from build123d import *

# Parameters (mm, degrees)
F1_W      = 129
F1_H      = 100.5
F1_W_2    = 127
F1_H_2    = 98.5
F2_DEPTH  = 6
F3_W      = 129
F3_H      = 100.5
F3_W_2    = 127
F3_H_2    = 90.5
F4_DEPTH  = 22
F6_DEPTH  = 17
F7_R      = 1.4
F8_DEPTH  = 7.9
F9_R      = 1.4
F10_DEPTH = 5
F11_W     = 127
F11_H     = 98.5
F11_W_2   = 115
F11_H_2   = 86
F12_DEPTH = 5


with BuildPart() as f2:
    # F1 (on Front) → F2 (new body)
    with BuildSketch(Plane.XZ):
        with Locations((1, -2.75)):
            Rectangle(F1_W, F1_H)
        with Locations((1, -2.75)):
            Rectangle(F1_W_2, F1_H_2, mode=Mode.SUBTRACT)
    extrude(amount=F2_DEPTH)

    # F3 (on Front) → F4 (join)
    with BuildSketch(Plane.XZ):
        with Locations((1, -2.75)):
            Rectangle(F3_W, F3_H)
        with Locations((1, -2.75)):
            Rectangle(F3_W_2, F3_H_2, mode=Mode.SUBTRACT)
    extrude(amount=-F4_DEPTH)

    # F5 (on face) → F6 (join)
    with BuildSketch(Plane(origin=(0, 22, 0), x_dir=(-1, 0, 0), z_dir=(0, 1, 0))):
        Polygon((3.5, -66.5), (63.5, -66.5), (63.5, -53), (55.5, -53), (55.5, -61.5), (11.5, -61.5), (11.5, -53), (3.5, -53), align=None)
    extrude(amount=-F6_DEPTH)

    # F7 (on face) → F8 (cut)
    with BuildSketch(Plane.XY.offset(47.5)):
        with Locations((-27.5, 16.5)):
            Circle(F7_R)
        with Locations((31.5, 16.5)):
            Circle(F7_R)
    extrude(amount=-F8_DEPTH, mode=Mode.SUBTRACT)

    # F9 (on face) → F10 (cut)
    with BuildSketch(Plane(origin=(0, 0, -66.5), x_dir=(1, 0, 0), z_dir=(0, 0, -1))):
        with Locations((-27.5, -16.5)):
            Circle(F9_R)
    extrude(amount=-F10_DEPTH, mode=Mode.SUBTRACT)

    # F11 (on face) → F12 (join)
    with BuildSketch(Plane.XZ):
        with Locations((1, -2.75)):
            Rectangle(F11_W, F11_H)
        Rectangle(F11_W_2, F11_H_2, mode=Mode.SUBTRACT)
    extrude(amount=F12_DEPTH)


solid = f2.part
For this review, take the finished solid that the model builds, in its own axes (mm). A direction names the side the tool comes from. Give positions to 0.01 mm unless a question says otherwise; leave off trailing zeros. Loops run counter-clockwise (first coordinate to the right, second up) from the corner with the lowest first, then second, coordinate; pieces in that order, holes last. Notation, with made-up numbers: (17.25, 40) - (65.25, 40) arc R23 ccw to (65.25, 71) - close; hole circle Ø4 at (-35.5, -13.5). An arc over 180 degrees is marked (long way). Write each question's results on one line, items separated by ' | '.
(1) Take a section at D-D (z = -24.5). Give the boundary of the cut face in (x, y).
Conclusion:
outline: (-63.5, -6) - (-62.5, -6) - (-62.5, -5) - (-57.5, -5) - (-57.5, 0) - (-62.5, 0) - (-62.5, 22) - (-63.5, 22) - close; (57.5, -5) - (64.5, -5) - (64.5, -6) - (65.5, -6) - (65.5, 22) - (64.5, 22) - (64.5, 0) - (57.5, 0) - close
(2) For faces 1 (the cylindrical face through (-28.53, 15.55, -64.04)), 2 (the flat face through (-55.5, 14, -57)), 3 (the flat face through (0, 11, -48)), list the 3-axis set-ups (+Z, -Z, +X, -X, +Y, -Y) from which the entire face can be reached by the end or side of a thin tool; tool diameter is ignored.
Conclusion:
face 1: -Z | face 2: +Y, -Y | face 3: +Y
(3) Take a section at B-B (y = 16.5). Give the boundary of the cut face in (x, z), then the cut area to 4 significant figures.
Conclusion:
outline: (-63.5, -66.5) - (-28.9, -66.5) - (-28.9, -61.5) - (-55.5, -61.5) - (-55.5, -53) - (-11.5, -53) - (-11.5, -61.5) - (-26.1, -61.5) - (-26.1, -66.5) - (-3.5, -66.5) - (-3.5, -53) - (65.5, -53) - (65.5, 47.5) - (32.9, 47.5) - (32.9, 42.5) - (64.5, 42.5) - (64.5, -48) - (-62.5, -48) - (-62.5, 42.5) - (-28.9, 42.5) - (-28.9, 47.5) - (-63.5, 47.5) - close; (-26.1, 42.5) - (30.1, 42.5) - (30.1, 47.5) - (-26.1, 47.5) - close | area: 1,865 mm^2
(4) Draft analysis for pull direction Z (two halves, no side actions). For faces 4 (the flat face through (-11.5, 14, -57)), 5 (the cylindrical face through (-28.53, 17.45, 45.04)), 6 (the flat face through (-33, 14, -66.5)), state which applies: +Z half, -Z half, draft (parallel to the pull), parting line (faces both ways), or undercut.
Conclusion:
face 4: undercut | face 5: draft | face 6: -Z half
(5) Take a section at C-C (y = -3). Give the boundary of the cut face in (x, z).
Conclusion:
outline: (-63.5, -53) - (65.5, -53) - (65.5, 47.5) - (-63.5, 47.5) - close; hole (-57.5, -43) - (57.5, -43) - (57.5, 43) - (-57.5, 43) - close
(6) For line 1 along Z through (x, y) = (-53.5, 20); line 2 along Y through (x, z) = (-27.5, 46.45); line 3 along Z through (x, y) = (56, 12.75), list the stretches that pass through material, from the lowest coordinate up.
Conclusion:
line 1: -66.5 to -61.5, -53 to -48, 42.5 to 47.5 | line 2: -5 to 15.1, 17.9 to 22 | line 3: -53 to -48, 42.5 to 47.5
(7) For pin 1 Ø1.1 at (x, y) = (7, -5.5) entering from -Z, flat-tipped, find the tip position at first contact; note if it passes through.
Conclusion:
pin 1: z = -53
(8) Take a section at A-A (x = 31.5). Give the boundary of the cut face in (y, z).
Conclusion:
outline: (-6, -53) - (22, -53) - (22, -48) - (0, -48) - (0, -43) - (-5, -43) - (-5, -52) - (-6, -52) - close; (-6, 46.5) - (-5, 46.5) - (-5, 43) - (0, 43) - (0, 42.5) - (15.1, 42.5) - (15.1, 47.5) - (-6, 47.5) - close; (17.9, 42.5) - (22, 42.5) - (22, 47.5) - (17.9, 47.5) - close
